Model file for the job. Use its own axes, mm. A direction names the side the tool comes from. Give positions to 0.01 mm unless a question says otherwise; leave off trailing zeros. Write each loop counter-clockwise with the first axis right and the second up, starting at its lowest first coordinate (ties: lowest second). Pieces come first, ordered by that corner, then holes. Notation, with made-up numbers: (7, -13.5) - (35, -13.5) arc R10 ccw to (35, 3.5) - close; hole circle Ø6 at (44, 20.5). An arc over 180 degrees is marked (long way). One line per item, written item: value. Start each with the question number.
(1) Cut at C-C, the plane x = 0. List the corners of the cut face in (y, z).
(2) Cut at B-B, the plane z = 18. List the corners of the cut face in (x, y), and give its area (3 significant figures).
(3) Probe L1, parallel to X at y = -26, z = 16; L2, parallel to X at y = -8, z = 12.25; L3, parallel to Y at x = 15, z = 17.5. List the from-to ranges inside material, lowest first.
(4) Mould opens along Y. For faces 6 (the face through (-18.078, -11.347, 12.647)), 7 (the face through (22.5, -28, 12)), 8 (the face through (11.01, -12.53, 0.99)) say: pulls with the +Y half, pulls with the -Y half, needs draft (parallel to the pull), parting line crosses it, or undercut.
(5) Cut at A-A, the plane y = -52. List the corners of the cut face in (x, z).
(6) Drop flat-ended pins along their axis: P1, Ø6, axis at x = 9, y = -25, coming from the -Z side; P2, Ø2, axis at x = -11.5, z = 14, coming from the +Y side; P3, Ø10, axis at y = 9.5, z = 15, coming from the +X side; P4, Ø5, axis at x = -5.5, z = 6, coming from the -Y side. Give the stop position or say it passes through.
(7) 3-axis set-ups, long thin cutter, end or side, ignore diameter. For faces 1 (the face through (-15.4, -3, 1)), 2 (the face through (7.5, -38, 12)), 3 (the face through (8.5, -37.9, 1)), 4 (the face through (10.039, -12.255, 12.353)), 5 (the face through (10.99, -12.52, 23.99)): which of +Z, -Z, +X, -X, +Y, -Y reach the whole face in a straight line?
from build123d import *

# Parameters (mm, degrees)
F0_R         = 5
F1_DEPTH     = 25
F2_R         = 5
F3_R         = 2
F4_T1_DEPTH  = 13.9731886125
F4_T3_DEPTH  = 27.1080898313
F4_T5_DEPTH  = 55
F4_T7_DEPTH  = 42.5305187235
F4_T9_DEPTH  = 5
F4_T12_ANGLE = 137.0297160683
F4_T14_ANGLE = 180
F4_T16_ANGLE = 207.1471098896
F4_T18_ANGLE = 90
F4_T20_ANGLE = 90
F4_T24_ANGLE = 137.0297160683
F4_T26_ANGLE = 180
F4_T28_ANGLE = 207.1471098896
F4_T30_ANGLE = 90
F4_T32_ANGLE = 90


# Not quite as in the source:
# - a fillet or chamfer that OpenCascade refuses, or shapes differently, is made with other operations: its cross-section is extruded or revolved along the edge and cut away or added


with BuildPart() as f1:
    # F0 (on Top) → F1 (new body)
    with BuildSketch(Plane.XY):
        with BuildLine():
            ThreePointArc((7.5, -21.2132034356), (18.3711730709, -12.9903810568), (22.5, 0))
            ThreePointArc((22.5, 0), (-7.4888899158, 21.2171281711), (-17.5148024737, -14.1237988625))
            Line((-17.5148024737, -14.1237988625), (-12.5074012369, 3.5447022866))
            ThreePointArc((-12.5074012369, 3.5447022866), (1.7893831229, 12.8762614155), (13, 0))
            ThreePointArc((13, 0), (12.8762614155, -1.7893831229), (12.5074012369, -3.5447022866))
            Line((12.5074012369, -3.5447022866), (7.5, -21.2132034356))
        make_face()
        with BuildLine():
            Line((22.5, -60), (22.5, 0))
            ThreePointArc((22.5, 0), (18.3711730709, -12.9903810568), (7.5, -21.2132034356))
            Line((7.5, -21.2132034356), (7.5, -60))
            Line((7.5, -60), (22.5, -60))
        make_face()
        with Locations((15, -52)):
            Circle(F0_R, mode=Mode.SUBTRACT)
    extrude(amount=F1_DEPTH)

    # F2
    f2_edges = [f1.edges().sort_by_distance(p)[0] for p in [
        (22.5, -60, 12.5),
        (7.5, -60, 12.5),
    ]]
    fillet(f2_edges, radius=F2_R)

    # F3
    f3_edges = [f1.edges().sort_by_distance(p)[0] for p in [
        (-17.514802, -14.123799, 12.5),
    ]]
    fillet(f3_edges, radius=F3_R)

    # F4: chamfer of 2 on 22 edges, made by hand

    # F4_s2 → F4_t1 (cut)
    with BuildSketch(Plane(origin=(-3.8100610481, -13.4437135796, 0), x_dir=(0, 0, 1), z_dir=(0.2726694067, 0.9621077875, 0))):
        Polygon((23, -13), (25, -15), (25, -13), align=None)
        Polygon((0, -15), (2, -13), (0, -13), align=None)
    extrude(amount=F4_T1_DEPTH, mode=Mode.SUBTRACT)

    # F4_s4 → F4_t3 (cut)
    with BuildSketch(Plane(origin=(0, 0, 0), x_dir=(0, 0, 1), z_dir=(-0.2726694067, -0.9621077875, 0))):
        Polygon((23, -13), (25, -15), (25, -13), align=None)
        Polygon((0, -15), (2, -13), (0, -13), align=None)
    extrude(amount=F4_T3_DEPTH, mode=Mode.SUBTRACT)

    # F4_s6 → F4_t5 (cut)
    with BuildSketch(Plane.XZ):
        Polygon((22.5, 23), (20.5, 25), (22.5, 25), align=None)
        Polygon((20.5, 0), (22.5, 2), (22.5, 0), align=None)
    extrude(amount=F4_T5_DEPTH, mode=Mode.SUBTRACT)

    # F4_s8 → F4_t7 (cut)
    with BuildSketch(Plane.XZ.offset(12.4694812765)):
        Polygon((7.5, 23), (9.5, 25), (7.5, 25), align=None)
        Polygon((9.5, 0), (7.5, 2), (7.5, 0), align=None)
    extrude(amount=F4_T7_DEPTH, mode=Mode.SUBTRACT)

    # F4_s10 → F4_t9 (cut)
    with BuildSketch(Plane.YZ.offset(12.5)):
        Polygon((-60, 23), (-58, 25), (-60, 25), align=None)
        Polygon((-58, 0), (-60, 2), (-60, 0), align=None)
    extrude(amount=F4_T9_DEPTH, mode=Mode.SUBTRACT)

    # F4_s11 → F4_t12 (revolve, cut)
    with BuildSketch(Plane(origin=(-3.8100610481, -13.4437135796, 0), x_dir=(0, 0, 1), z_dir=(0.2726694067, 0.9621077875, 0))):
        Polygon((23, -13), (25, -15), (25, -13), align=None)
    revolve(axis=Axis((-18.2416778599, -9.3536724797, 25), (0, 0, -1)), revolution_arc=F4_T12_ANGLE, mode=Mode.SUBTRACT)

    # F4_s13 → F4_t14 (revolve, cut)
    with BuildSketch(Plane(origin=(0, 0, 0), x_dir=(0, 0, 1), z_dir=(-0.2726694067, -0.9621077875, 0))):
        Polygon((23, 13), (25, 15), (25, 13), align=None)
    revolve(axis=Axis((0, 0, 25), (0, 0, -1)), revolution_arc=F4_T14_ANGLE, mode=Mode.SUBTRACT)

    # F4_s15 → F4_t16 (revolve, cut)
    with BuildSketch(Plane.XZ):
        Polygon((22.5, 23), (20.5, 25), (22.5, 25), align=None)
    revolve(axis=Axis((0, 0, 25), (0, 0, 1)), revolution_arc=F4_T16_ANGLE, mode=Mode.SUBTRACT)

    # F4_s17 → F4_t18 (revolve, cut)
    with BuildSketch(Plane.YZ.offset(17.5)):
        Polygon((-60, 23), (-58, 25), (-60, 25), align=None)
    revolve(axis=Axis((17.5, -55, 25), (0, 0, 1)), revolution_arc=F4_T18_ANGLE, mode=Mode.SUBTRACT)

    # F4_s19 → F4_t20 (revolve, cut)
    with BuildSketch(Plane.XZ.offset(55)):
        Polygon((7.5, 23), (9.5, 25), (7.5, 25), align=None)
    revolve(axis=Axis((12.5, -55, 25), (0, 0, 1)), revolution_arc=F4_T20_ANGLE, mode=Mode.SUBTRACT)

    # F4_s21 → F4_t22 (revolve, cut)
    with BuildSketch(Plane.XZ.offset(52)):
        Polygon((20, 23), (22, 25), (20, 25), align=None)
    revolve(axis=Axis((15, -52, 25), (0, 0, 1)), mode=Mode.SUBTRACT)

    # F4_s23 → F4_t24 (revolve, cut)
    with BuildSketch(Plane(origin=(-3.8100610481, -13.4437135796, 0), x_dir=(0, 0, 1), z_dir=(0.2726694067, 0.9621077875, 0))):
        Polygon((0, -15), (2, -13), (0, -13), align=None)
    revolve(axis=Axis((-18.2416778599, -9.3536724797, 0), (0, 0, -1)), revolution_arc=F4_T24_ANGLE, mode=Mode.SUBTRACT)

    # F4_s25 → F4_t26 (revolve, cut)
    with BuildSketch(Plane(origin=(0, 0, 0), x_dir=(0, 0, 1), z_dir=(-0.2726694067, -0.9621077875, 0))):
        Polygon((0, 15), (2, 13), (0, 13), align=None)
    revolve(axis=Axis((0, 0, 0), (0, 0, -1)), revolution_arc=F4_T26_ANGLE, mode=Mode.SUBTRACT)

    # F4_s27 → F4_t28 (revolve, cut)
    with BuildSketch(Plane.XZ):
        Polygon((20.5, 0), (22.5, 2), (22.5, 0), align=None)
    revolve(axis=Axis((0, 0, 0), (0, 0, 1)), revolution_arc=F4_T28_ANGLE, mode=Mode.SUBTRACT)

    # F4_s29 → F4_t30 (revolve, cut)
    with BuildSketch(Plane.YZ.offset(17.5)):
        Polygon((-58, 0), (-60, 2), (-60, 0), align=None)
    revolve(axis=Axis((17.5, -55, 0), (0, 0, 1)), revolution_arc=F4_T30_ANGLE, mode=Mode.SUBTRACT)

    # F4_s31 → F4_t32 (revolve, cut)
    with BuildSketch(Plane.XZ.offset(55)):
        Polygon((9.5, 0), (7.5, 2), (7.5, 0), align=None)
    revolve(axis=Axis((12.5, -55, 0), (0, 0, 1)), revolution_arc=F4_T32_ANGLE, mode=Mode.SUBTRACT)

    # F4_s33 → F4_t34 (revolve, cut)
    with BuildSketch(Plane.XZ.offset(52)):
        Polygon((22, 0), (20, 2), (20, 0), align=None)
    revolve(axis=Axis((15, -52, 0), (0, 0, 1)), mode=Mode.SUBTRACT)


solid = f1.part
Answers follow:
1. outline: (13, 2) - (15, 0) - (20.5, 0) - (22.5, 2) - (22.5, 23) - (20.5, 25) - (15, 25) - (13, 23) - close
2. outline: (-20.02, -10.27) arc R2 ccw to (-16.32, -9.9) - (-12.51, 3.54) arc R13 cw to (12.51, -3.54) - (7.5, -21.21) - (7.5, -55) arc R5 ccw to (12.5, -60) - (17.5, -60) arc R5 ccw to (22.5, -55) - (22.5, 0) arc R22.5 ccw (long way) to start; hole circle Ø10 at (15, -52)
2. area: 1,350 mm²
3. L1: x = 7.5 to 22.5
3. L2: x = -21.03 to -15.78, 11.24 to 22.5
3. L3: y = -60 to -57, -47 to 16.77
4. face 6: pulls with the -Y half
4. face 7: needs draft
4. face 8: undercut
5. outline: (7.5, 2) - (8.75, 0.75) - (10, 2) - (10, 23) - (8.75, 24.25) - (7.5, 23) - close; (20, 2) - (21.25, 0.75) - (22.5, 2) - (22.5, 23) - (21.25, 24.25) - (20, 23) - close
6. P1: stops at z = 0
6. P2: stops at y = 19.9
6. P3: stops at x = 22.05
6. P4: stops at y = 10.25
7. face 1: -Z, -Y
7. face 2: +Z, -Z, -X, -Y
7. face 3: -Z, -X, -Y
7. face 4: +Z, -Z
7. face 5: +Z
